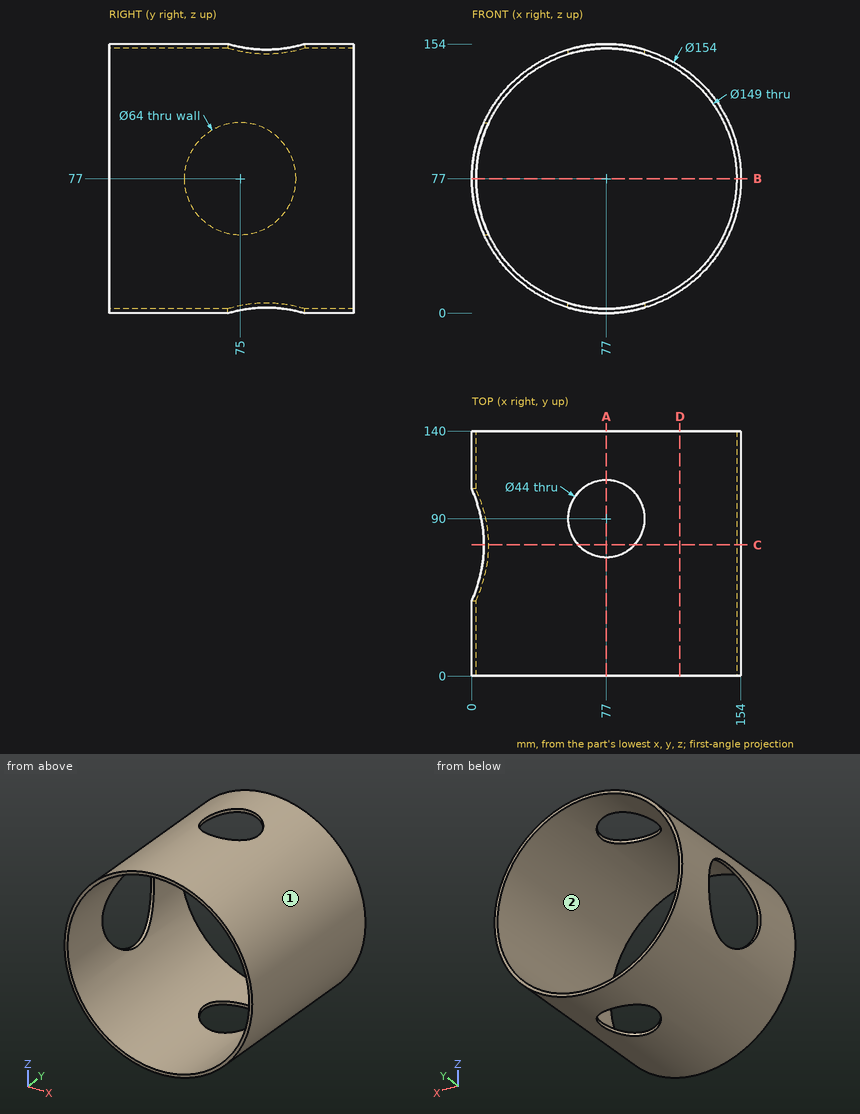
Geometry: see drawing. Coordinates: mm, zero at the bounding-box minimum. Give positions to 0.01 mm unless a question says otherwise; leave off trailing zeros. Loops run counter-clockwise (first coordinate to the right, second up) from the corner with the lowest first, then second, coordinate; pieces in that order, holes last. Notation, with made-up numbers: M 8.25,-36.5 L 16.25,-36.5 A34 ccw 16.25,-5.5 Z; hole C 67.5,28 d2. An arc over 180 degrees is marked long. Answer as CSV lines item,"result". Start each with the question number.
1. Pull-direction query (X, two-part tool) for the marked faces 1 and 2; classes: released by +X, released by -X, zero draft, split by the parting line, or undercut.
2. Section A-A on x = 77. Return loops of the section in (y, z), plus the area to 3 significant figures.
3. Line query: L1, parallel to Z at x = 13, y = 39; L2, parallel to Z at x = 71, y = 116.5; L3, parallel to X at y = 6, z = 125. Output: solid intervals per line, ascending.
4. Pin query (flat end, axial travel): P1, Ø5, axis at y = 125.5, z = 123.5, coming from the +X side; P2, Ø1, axis at x = 23.5, z = 126, coming from the +Y side; P3, Ø5, axis at y = 88.5, z = 83, coming from the -X side; P4, Ø3, axis at y = 69, z = 70.5, coming from the +X side. Return the tip coordinate at first contact, or that it passes through.
5. Section D-D on x = 119. Return loops of the section in (y, z).
6. Section C-C on y = 75. Return loops of the section in (x, z), plus the area to 3 significant figures.
7. Section B-B on z = 77. Return loops of the section in (x, y), plus the area to 3 significant figures.
Computed values:
1,face 1,"split by the parting line"
1,face 2,"undercut"
2,outline,"M 0,0 L 68,0 L 68,2.5 L 0,2.5 Z; M 0,151.5 L 68,151.5 L 68,154 L 0,154 Z; M 112,0 L 140,0 L 140,2.5 L 112,2.5 Z; M 112,151.5 L 140,151.5 L 140,154 L 112,154 Z"
2,area,"480 mm²"
3,L1,"z = 34.19 to 38.87, 115.13 to 119.81"
3,L2,"z = 0.23 to 2.74, 151.26 to 153.77"
3,L3,"x = 16.79 to 20.02, 133.98 to 137.21"
4,P1,"stops at x = 140.19"
4,P2,"passes through"
4,P3,"stops at x = 151.01"
4,P4,"stops at x = 153.84"
5,outline,"M 0,12.46 L 140,12.46 L 140,15.47 L 0,15.47 Z; M 0,138.53 L 140,138.53 L 140,141.54 L 0,141.54 Z"
6,outline,"M 6.96,45 A77 ccw 60.91,1.7 L 60.91,4.26 A74.5 cw 9.72,45 Z; M 6.96,109 L 9.72,109 A74.5 cw 60.91,149.74 L 60.91,152.3 A77 ccw Z; M 93.09,1.7 A77 ccw 93.09,152.3 L 93.09,149.74 A74.5 cw 93.09,4.26 Z"
6,area,"863 mm²"
7,outline,"M 0,0 L 2.5,0 L 2.5,43 L 0,43 Z; M 0,107 L 2.5,107 L 2.5,140 L 0,140 Z; M 151.5,0 L 154,0 L 154,140 L 151.5,140 Z"
7,area,"540 mm²"
